```python
from build123d import *

# Parameters (mm, degrees)
BOSS_EXTRUDE1_DEPTH              = 3.175
F_10_0_1935_DIAMETER_HOLE1_D     = 4.9149
F_10_0_1935_DIAMETER_HOLE1_DEPTH = 19.001994
F_10_0_1935_DIAMETER_HOLE1_TIP   = 1.476584928
SKETCH4_R                        = 1.5875
CUT_EXTRUDE1_DEPTH               = 59.987451342


with BuildPart() as part:
    # Sketch1 → Boss-Extrude1 (new body)
    with BuildSketch(Plane(origin=(0, 0, 0), x_dir=(0, 0, -1), z_dir=(1, 0, 0))):
        with BuildLine():
            Line((1.5875, 46.219867315), (1.5875, 36.694867315))
            Line((1.5875, 36.694867315), (-1.5875, 36.694867315))
            Line((-1.5875, 36.694867315), (-1.5875, 46.219867315))
            ThreePointArc((-1.5875, 46.219867315), (-12.594751518, 43.710922642), (-21.42746878, 36.679742434))
            Line((-21.42746878, 36.679742434), (-25.39243756, 31.719750239))
            ThreePointArc((-25.39243756, 31.719750239), (-33.651945283, 16.80623652), (-36.5125, 0))
            Line((-36.5125, 0), (-36.5125, -19.05))
            Line((-36.5125, -19.05), (-14.2875, -19.05))
            Line((-14.2875, -19.05), (-14.2875, 0))
            ThreePointArc((-14.2875, 0), (0, 14.2875), (14.2875, 0))
            Line((14.2875, 0), (14.2875, -19.05))
            Line((14.2875, -19.05), (36.5125, -19.05))
            Line((36.5125, -19.05), (36.5125, 0))
            ThreePointArc((36.5125, 0), (33.651945283, 16.80623652), (25.39243756, 31.719750239))
            Line((25.39243756, 31.719750239), (21.42746878, 36.679742434))
            ThreePointArc((21.42746878, 36.679742434), (12.594751518, 43.710922642), (1.5875, 46.219867315))
        make_face()
    extrude(amount=BOSS_EXTRUDE1_DEPTH)

    # #10 (0.1935) Diameter Hole1
    with Locations(Plane.ZY):
        with Locations((-25.4, -6.35), (25.4, -6.35)):
            Hole(F_10_0_1935_DIAMETER_HOLE1_D / 2, depth=F_10_0_1935_DIAMETER_HOLE1_DEPTH)
            with Locations((0, 0, -(F_10_0_1935_DIAMETER_HOLE1_DEPTH + F_10_0_1935_DIAMETER_HOLE1_TIP / 2))):  # 118° drill point
                Cone(0, F_10_0_1935_DIAMETER_HOLE1_D / 2, F_10_0_1935_DIAMETER_HOLE1_TIP, mode=Mode.SUBTRACT)

    # Sketch4 → Cut-Extrude1 (cut, through all)
    with BuildSketch(Plane(origin=(3.175, 0, 0), x_dir=(0, 0, -1), z_dir=(1, 0, 0))):
        with Locations((-19.842621022, 5.0165)):
            Circle(SKETCH4_R)
        with Locations((0, 20.8915)):
            Circle(SKETCH4_R)
        with Locations((19.842621022, 5.0165)):
            Circle(SKETCH4_R)
    extrude(amount=-CUT_EXTRUDE1_DEPTH, mode=Mode.SUBTRACT)


solid = part.part
```
Check sheet for the modelled part. Datum: model origin and axes. Units: mm. A direction names the side the tool comes from. Round coordinates to 2 decimals unless told otherwise and drop trailing zeros. Order: outer loops, then holes, each group sorted by start corner. A loop starts at its lowest first (then second) coordinate and runs counter-clockwise, first axis right, second up. Notation, with made-up numbers: (76.5, 20.25) - (106.5, 20.25) arc R32 cw to (106.5, 59.25) - close; hole circle Ø6 at (6, 64). An arc over 180 degrees is marked (long way). Write item = value, one per line.
Q1. Section check A-A (y = -11.5). Record the boundary of the cut face in (x, z) (1 decimal), and give its area (3 significant figures).
Computed:
outline = (0, -36.5) - (3.2, -36.5) - (3.2, -14.3) - (0, -14.3) - close; (0, 14.3) - (3.2, 14.3) - (3.2, 36.5) - (0, 36.5) - close
area = 141 mm^2
Q2. Section check B-B (z = 0). Record the boundary of the cut face in (x, y) (1 decimal), and give its area (3 significant figures).
Computed:
outline = (0, 14.3) - (3.2, 14.3) - (3.2, 19.3) - (0, 19.3) - close; (0, 22.5) - (3.2, 22.5) - (3.2, 36.7) - (0, 36.7) - close
area = 61.1 mm^2
Q3. Thickness scan on line 1 along Z through (x, y) = (0.7, -9); line 2 along Y through (x, z) = (1.45, 0); line 3 along Z through (x, y) = (1.5, 40). Record the ranges inside material, lowest first.
Computed:
line_1 = -36.51 to -14.29, 14.29 to 36.51
line_2 = 14.29 to 19.3, 22.48 to 36.69
line_3 = -18.24 to -1.59, 1.59 to 18.24
Q4. Tool access check on faces 4 (the face through (1.61, -4.69, 27.21)), 5 (the face through (2, -10, 14.288)). Record the directions out of +Z, -Z, +X, -X, +Y, -Y that give a thin tool (end or side, any length) a straight path to the whole face; none if there is none.
Computed:
face_4 = +X, -X
face_5 = +X, -X, -Y
Q5. Go/stop test with flat-tipped pins: pin 1 (5 mm diameter, centred on y = 5.02, z = 19.84, fed in from +X) (3 decimals); pin 2 (4 mm diameter, centred on y = -6.35, z = -25.4, fed in from -X); pin 3 (1 mm diameter, centred on x = 2, z = -0.5, fed in from +Y). Record where each tip stops, or that it passes through.
Computed:
pin_1 = 3.175
pin_2 = through
pin_3 = 36.69
Q6. Draft check along Y on faces 1 (the face through (2, -9, 36.512)), 2 (the face through (1.61, 4.41, -21.31)), 3 (the face through (1.565, 34.234, 23.382)). Enter one of: pulls with the +Y half, pulls with the -Y half, needs draft (parallel to the pull), parting line crosses it, or undercut.
Computed:
face_1 = needs draft
face_2 = undercut
face_3 = pulls with the +Y half
Q7. Section check D-D (z = -7.5). Record the boundary of the cut face in (x, y) (3 decimals).
Computed:
outline = (0, 12.161) - (3.175, 12.161) - (3.175, 45.522) - (0, 45.522) - close
Q8. Section check C-C (x = 1.55). State how many separate pieces and enclosed holes the cut face has, and give its area (3 significant figures).
Computed:
separate_pieces = 1
enclosed_holes = 5
area = 3,050 mm^2
